```python
from build123d import *

# Parameters (mm, degrees)
F0_R     = 3.175
F1_DEPTH = 6.35


# Not quite as in the source:
# - a feature names something its author has since deleted; it is built from what else it names


with BuildPart() as f1:
    # F0 (on Top) → F1 (new body, symmetric)
    with BuildSketch(Plane.XY):
        with BuildLine():
            Line((245.237, 38.1), (-245.237, 38.1))
            Line((-245.237, 38.1), (-245.237, -38.1))
            Line((-245.237, -38.1), (245.237, -38.1))
            ThreePointArc((245.237, -38.1), (274.8200168552, -34.2053219448), (302.387, -22.7867036526))
            Line((302.387, -22.7867036526), (416.687, 43.2044321158))
            ThreePointArc((416.687, 43.2044321158), (430.6325678842, 95.25), (378.587, 109.1955678842))
            Line((378.587, 109.1955678842), (321.437, 76.2))
            Line((321.437, 76.2), (264.287, 43.2044321158))
            ThreePointArc((264.287, 43.2044321158), (255.0980056184, 39.3982260184), (245.237, 38.1))
        make_face()
        with Locations((-207.137, 0)):
            Circle(F0_R, mode=Mode.SUBTRACT)
        with BuildLine():
            ThreePointArc((394.887369343, 74.6125), (396.8152495318, 79.2668144985), (400.812, 76.2))
            ThreePointArc((400.812, 76.2), (398.4587504682, 73.1331855015), (394.887369343, 74.6125))
        make_face(mode=Mode.SUBTRACT)
    extrude(amount=F1_DEPTH, both=True)


solid = f1.part
```
Verification items for the finished model (mm, model axes). A direction names the side the tool comes from. Round coordinates to 2 decimals unless told otherwise and drop trailing zeros. Order: outer loops, then holes, each group sorted by start corner. A loop starts at its lowest first (then second) coordinate and runs counter-clockwise, first axis right, second up. Notation, with made-up numbers: (83.5, 18) -> (114.5, 18) arc R7 ccw to (114.5, 22) -> close; hole circle Ø5 at (80.5, 12.25). An arc over 180 degrees is marked (long way). Put each result on its own line as item: value. Start each with the question number.
(1) Section check B-B (x = 60.5). Enter the section's corners in (y, z), then the cut area to 3 significant figures.
(2) Section check A-A (z = 4.25). State how many separate pieces and enclosed holes the cut face has, then the cut area to 3 significant figures.
(3) Tool access check on faces 1 (the face through (358.74, 9.75, 0.09)), 2 (the face through (3, 38.1, 0)). Record the directions out of +Z, -Z, +X, -X, +Y, -Y that give a thin tool (end or side, any length) a straight path to the whole face; none if there is none.
(4) Depth check by flat-ended pin: pin 1 Ø1.5 at (x, z) = (99.5, 1.5) entering from +Y; pin 2 Ø5 at (y, z) = (74, -2) entering from -X; pin 3 Ø5 at (x, y) = (397.637, 76.2) entering from +Z; pin 4 Ø2 at (x, z) = (343.5, -2.5) entering from -Y. Enter the tip coordinate at first touch or a pass-through.
(5) Material ranges on line 1 along Y through (x, z) = (-161.5, 2); line 2 along X through (y, z) = (76.2, -4); line 3 along X through (y, z) = (36, -3.75), recorded low to high.
(6) Section check C-C (x = 311). Enter the section's corners in (y, z), then the cut area to 3 significant figures.
Completed:
1. outline: (-38.1, -6.35) -> (38.1, -6.35) -> (38.1, 6.35) -> (-38.1, 6.35) -> close
1. area: 968 mm2
2. separate pieces: 1
2. enclosed holes: 2
2. area: 52,700 mm2
3. face 1: +Z, -Z, +X, -Y
3. face 2: +Z, -Z, -X, +Y
4. pin 1: stops at y = 38.1
4. pin 2: stops at x = 313.3
4. pin 3: passes through
4. pin 4: stops at y = 0.37
5. line 1: y = -38.1 to 38.1
5. line 2: x = 321.44 to 394.46, 400.81 to 435.74
5. line 3: x = -245.24 to 404.21
6. outline: (-17.81, -6.35) -> (70.17, -6.35) -> (70.17, 6.35) -> (-17.81, 6.35) -> close
6. area: 1,120 mm2
